from build123d import *

# Parameters (mm, degrees)
F0_W     = 50
F0_H     = 40
F1_DEPTH = 20
F2_W     = 30
F2_H     = 20
F3_DEPTH = 20
F5_DEPTH = 20


with BuildPart() as f1:
    # F0 (on Top) → F1 (new body)
    with BuildSketch(Plane.XY):
        with Locations((25, 20)):
            Rectangle(F0_W, F0_H)
    extrude(amount=F1_DEPTH)

    # F2 (on face) → F3 (cut)
    with BuildSketch(Plane.XY.offset(20)):
        with Locations((25, 20)):
            Rectangle(F2_W, F2_H)
    extrude(amount=-F3_DEPTH, mode=Mode.SUBTRACT)

    # F4 (on face) → F5 (join)
    with BuildSketch(Plane.XZ.offset(-30)):
        Polygon((20, 0), (10, 20), (10, 0), align=None)
    extrude(amount=F5_DEPTH)


solid = f1.part
Geometry: final body of the model. Coordinates: model frame, mm. A direction names the side the tool comes from. Give positions to 0.01 mm unless a question says otherwise; leave off trailing zeros. Write each loop counter-clockwise with the first axis right and the second up, starting at its lowest first coordinate (ties: lowest second). Pieces come first, ordered by that corner, then holes. Notation, with made-up numbers: (57.25, -8) -> (115.25, -8) arc R22 cw to (115.25, 29) -> close; hole circle Ø5 at (62, -37.75). An arc over 180 degrees is marked (long way). Answer in a Markdown table with one row per item.
(1) Section query B-B on y = 15.5. Return loops of the section in (x, z).
Answers below:
| item | result |
|---|---|
| outline | (0, 0) -> (20, 0) -> (10, 20) -> (0, 20) -> close; (40, 0) -> (50, 0) -> (50, 20) -> (40, 20) -> close |
(2) Draft query along Y for faces 4 (the flat face through (28, 10, 10)), 5 (the flat face through (25, 40, 10)), 6 (the flat face through (25, 0, 10)), 7 (the flat face through (50, 20, 10)). Return one class per face: +Y half, -Y half, draft (parallel to the pull), parting line (faces both ways), or undercut.
Answers below:
| item | result |
|---|---|
| face 4 | undercut |
| face 5 | +Y half |
| face 6 | -Y half |
| face 7 | draft |
(3) Section query C-C on z = 14. Return loops of the section in (x, y), then the cut area to 3 significant figures.
Answers below:
| item | result |
|---|---|
| outline | (0, 0) -> (50, 0) -> (50, 40) -> (0, 40) -> close; hole (13, 10) -> (40, 10) -> (40, 30) -> (13, 30) -> close |
| area | 1,460 mm^2 |
(4) Section query D-D on z = 4.5. Return loops of the section in (x, y), then the cut area to 4 significant figures.
Answers below:
| item | result |
|---|---|
| outline | (0, 0) -> (50, 0) -> (50, 40) -> (0, 40) -> close; hole (17.75, 10) -> (40, 10) -> (40, 30) -> (17.75, 30) -> close |
| area | 1,555 mm^2 |
(5) Ray query, line 1 along Y through (x, z) = (36, 5); line 2 along X through (y, z) = (20, 11); line 3 along X through (y, z) = (28.5, 5). Return the intervals inside material, ascending. Write a range as [from, to].
Answers below:
| item | result |
|---|---|
| line 1 | [0, 10], [30, 40] |
| line 2 | [0, 14.5], [40, 50] |
| line 3 | [0, 17.5], [40, 50] |
(6) Set-up query: faces 1 (the flat face through (28, 30, 10)), 2 (the flat face through (0, 20, 10)), 3 (the flat face through (40, 20, 10)). Return all of +Z, -Z, +X, -X, +Y, -Y with unobstructed straight access to the full face (end or side cutting, diameter ignored); none if empty.
Answers below:
| item | result |
|---|---|
| face 1 | +Z |
| face 2 | +Z, -Z, -X, +Y, -Y |
| face 3 | +Z, -Z |
(7) Section query A-A on x = 37.5. Return loops of the section in (y, z), then the cut area to 3 significant figures.
Answers below:
| item | result |
|---|---|
| outline | (0, 0) -> (10, 0) -> (10, 20) -> (0, 20) -> close; (30, 0) -> (40, 0) -> (40, 20) -> (30, 20) -> close |
| area | 400 mm^2 |
